Geometry check sheet. Reference: the model listing, model coordinates, mm. Face numbers are marked on the shaded views. A direction names the side the tool comes from. Round coordinates to 2 decimals unless told otherwise and drop trailing zeros. Order: outer loops, then holes, each group sorted by start corner. A loop starts at its lowest first (then second) coordinate and runs counter-clockwise, first axis right, second up.
(1) Sectioned sample at A-A (y = 2.5). Record the boundary of the cut face in (x, z) (1 decimal), plus the area to 3 significant figures.
(2) Go/stop test with flat-tipped pins: pin 1 (3 mm diameter, centred on x = -13, y = 16, fed in from +Z) (3 decimals); pin 2 (3.5 mm diameter, centred on x = -52.06, z = 36.91, fed in from -Y); pin 3 (8 mm diameter, centred on y = 3, z = 34.5, fed in from -X); pin 4 (12.5 mm diameter, centred on x = -39, z = 26, fed in from +Y) (3 decimals). Record where each tip stops, or that it passes through.
(3) Sectioned sample at C-C (y = 23.5). Record the boundary of the cut face in (x, z) (3 decimals), plus the area to 3 significant figures.
(4) Set-up check for the marked faces 1 and 2: record each of +Z, -Z, +X, -X, +Y, -Y from which the full face is reachable in a straight line by a thin tool's end or side.
(5) Sectioned sample at B-B (x = -34.5). Record the boundary of the cut face in (y, z) (3 decimals).
(6) Sectioned sample at D-D (x = -19.5). Record the boundary of the cut face in (y, z) (3 decimals), plus the area to 3 significant figures.
(7) Material ranges on line 1 along Y through (x, z) = (-27, 23.5) (3 decimals); line 2 along Z through (x, y) = (-8, 9.75) (3 decimals); line 3 along Z through (x, y) = (-61, 2.25), recorded low to high.
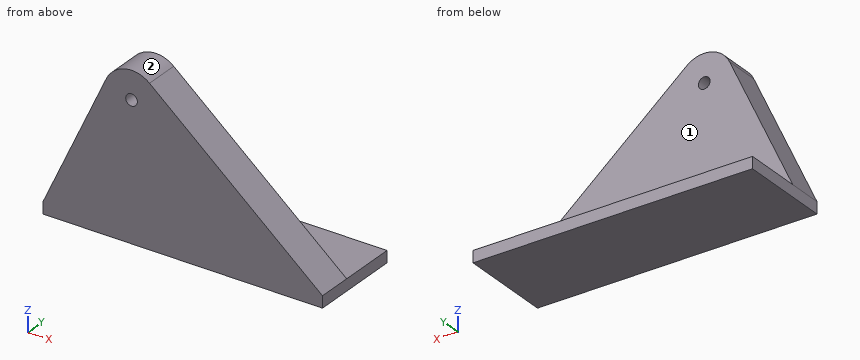
from build123d import *

# Parameters (mm, degrees)
SKETCH1_W               = 76.2
SKETCH1_H               = 25.4
BOSS_EXTRUDE1_DEPTH     = 3.175
BOSS_EXTRUDE2_DEPTH     = 9.525
CUT_EXTRUDE1_DEPTH      = 90.67460564
CUT_EXTRUDE1_DEPTH_BACK = 9.525
SKETCH3_R               = 1.5875


with BuildPart() as part:
    # Sketch1 → Boss-Extrude1 (new body)
    with BuildSketch(Plane.XY):
        with Locations((-38.1, 12.7)):
            Rectangle(SKETCH1_W, SKETCH1_H)
    extrude(amount=BOSS_EXTRUDE1_DEPTH)

    # Sketch2 → Boss-Extrude2 (add)
    with BuildSketch(Plane(origin=(0, 0, 0), x_dir=(-1, 0, 0), z_dir=(0, -1, 0))):
        with BuildLine():
            Line((0, 0), (76.2, 0))
            Line((76.2, 0), (76.2, -3.175))
            Line((76.2, -3.175), (58.966607548, -40.132129378))
            ThreePointArc((58.966607548, -40.132129378), (53.709812069, -44.351153797), (47.162500625, -42.74903688))
            Line((47.162500625, -42.74903688), (0, -3.175))
            Line((0, -3.175), (0, 0))
        make_face()
    extrude(amount=-BOSS_EXTRUDE2_DEPTH)

    # Sketch3 → Cut-Extrude1 (cut, two sides: drawn at the far end of the back side and taken through both)
    with BuildSketch(Plane(origin=(0, 9.525, 0), x_dir=(1, 0, 0), z_dir=(0, 1, 0)).offset(-CUT_EXTRUDE1_DEPTH_BACK)):
        with Locations(Location((-52.060542211, -36.911778223, 0), (0, 0, 180))):
            Circle(SKETCH3_R)
    extrude(amount=CUT_EXTRUDE1_DEPTH + CUT_EXTRUDE1_DEPTH_BACK, mode=Mode.SUBTRACT)


solid = part.part
Answer below:
1. outline: (-76.2, 0) - (0, 0) - (0, 3.2) - (-47.2, 42.7) arc R7.6 ccw to (-59, 40.1) - (-76.2, 3.2) - close; hole circle Ø3.2 at (-52.1, 36.9)
1. area: 1,960 mm2
2. pin 1: stops at z = 3.175
2. pin 2: stops at y = 0
2. pin 3: stops at x = -63.46
2. pin 4: stops at y = 9.525
3. outline: (-76.2, 0) - (0, 0) - (0, 3.175) - (-76.2, 3.175) - close
3. area: 242 mm2
4. face 1: +Z, +X, -X, +Y
4. face 2: +Z, +Y, -Y
5. outline: (0, 0) - (25.4, 0) - (25.4, 3.175) - (9.525, 3.175) - (9.525, 32.124) - (0, 32.124) - close
6. outline: (0, 0) - (25.4, 0) - (25.4, 3.175) - (9.525, 3.175) - (9.525, 19.537) - (0, 19.537) - close
6. area: 236 mm2
7. line 1: y = 0 to 9.525
7. line 2: z = 0 to 3.175
7. line 3: z = 0 to 35.77
